from build123d import *


with BuildPart() as part:
    # Esquisse1 → Base-Révolution (revolve)
    with BuildSketch(Plane.XY, mode=Mode.PRIVATE) as base_r_volution_sk:
        with BuildLine():
            Line((0, 0), (0, -0.650445183))
            ThreePointArc((0, -0.650445183), (-2.521065198, -0.487151674), (-5, 0))
            Line((-5, 0), (-5, 1))
            Line((-5, 1), (-4, 1))
            Line((-4, 1), (-4, 8))
            Line((-4, 8), (-8, 8))
            Line((-8, 8), (-8, 10))
            Line((-8, 10), (-4, 10))
            Line((-4, 10), (-4, 15))
            Line((-4, 15), (-5, 15))
            Line((-5, 15), (-5, 16))
            ThreePointArc((-5, 16), (-2.53207593, 16.601354724), (0, 16.803513576))
            Line((0, 16.803513576), (0, 16))
            Line((0, 16), (0, 0))
        make_face()
    revolve(base_r_volution_sk.sketch.rotate(Axis((0, 0, 0), (0, 1, 0)), 270), axis=Axis((0, 0, 0), (0, 1, 0)))


solid = part.part
The listing builds one solid part. Answer for the finished solid, in the listing's coordinates (mm). A direction names the side the tool comes from. Give positions to 0.01 mm unless a question says otherwise; leave off trailing zeros. Loops run counter-clockwise (first coordinate to the right, second up) from the corner with the lowest first, then second, coordinate; pieces in that order, holes last. Notation, with made-up numbers: M 61,-16 L 85,-16 A17 cw 85,12 Z; hole C -11,63.25 d7. An arc over 180 degrees is marked long. Answer as CSV lines item,"result".
Item 1: The part is cut by section C-C (y = 8.75). Give the vertices of the cut face in (x, z).
Values follow:
outline,"C 0,0 d16"
Item 2: The mould has two halves that part along Y. Classify faces 1 (the cylindrical face through (3.905, 12.535, 0.867)), 2 (the cylindrical face through (4.88, 15.51, 1.08)): released by +Y, released by -Y, zero draft, split by the parting line, or undercut.
Values follow:
face 1,"undercut"
face 2,"zero draft"
Item 3: The part is cut by section A-A (z = 0). Give the vertices of the cut face in (x, y).
Values follow:
outline,"M -8,8 L -4,8 L -4,1 L -5,1 L -5,0 A19.54 ccw 5,0 L 5,1 L 4,1 L 4,8 L 8,8 L 8,10 L 4,10 L 4,15 L 5,15 L 5,16 A15.96 ccw -5,16 L -5,15 L -4,15 L -4,10 L -8,10 Z"
Item 4: The part is cut by section D-D (x = 0). Give the vertices of the cut face in (y, z).
Values follow:
outline,"M 0,-5 L 1,-5 L 1,-4 L 8,-4 L 8,-8 L 10,-8 L 10,-4 L 15,-4 L 15,-5 L 16,-5 A15.96 ccw 16,5 L 15,5 L 15,4 L 10,4 L 10,8 L 8,8 L 8,4 L 1,4 L 1,5 L 0,5 A19.54 ccw Z"
Item 5: Straight lines are drawn through the part: line 1 along Y through (x, z) = (4.5, -3.5); line 2 along Z through (x, y) = (-0.5, 11.5); line 3 along X through (y, z) = (8.5, 4.25). For each, find the intervals that lie inside material, in ascending order. Write a range as [from, to].
Values follow:
line 1,"y = [8, 10]"
line 2,"z = [-3.97, 3.97]"
line 3,"x = [-6.78, 6.78]"
Item 6: Given pin 1 Ø5 at (y, z) = (6, 1.5) entering from +X; pin 2 Ø6 at (x, z) = (-2.5, -6.5) entering from -Y; pin 3 Ø2 at (y, z) = (9.5, 4) entering from -X; pin 4 Ø5 at (x, z) = (-5, 0) entering from +Y, each flat-ended and moving along its own axis, determine where each tip first touches the part or whether it passes through.
Values follow:
pin 1,"stops at x = 8"
pin 2,"stops at y = -0.24"
pin 3,"stops at x = -7.42"
pin 4,"stops at y = 16.61"
Item 7: Which of the six approach directions +Z, -Z, +X, -X, +Y, -Y give full straight-line access (tool end or side, diameter ignored) to faces 3 (the cylindrical face through (4.88, 0.51, 1.08)), 4 (the cylindrical face through (3.905, 4.549, 0.867)), 5 (the cylindrical face through (7.81, 9.01, 1.73))?
Values follow:
face 3,"-Y"
face 4,"none"
face 5,"+Y, -Y"
Item 8: The part is cut by section B-B (x = -1.75). Give the vertices of the cut face in (y, z), and give its area (3 significant figures).
Values follow:
outline,"M 0,-4.68 L 1,-4.68 L 1,-3.6 L 8,-3.6 L 8,-7.81 L 10,-7.81 L 10,-3.6 L 15,-3.6 L 15,-4.68 L 16,-4.68 A15.86 ccw 16,4.68 L 15,4.68 L 15,3.6 L 10,3.6 L 10,7.81 L 8,7.81 L 8,3.6 L 1,3.6 L 1,4.68 L 0,4.68 A19.46 ccw Z"
area,"144 mm^2"
